The listing builds one solid part. Answer for the finished solid, in the listing's coordinates (mm). A direction names the side the tool comes from. Give positions to 0.01 mm unless a question says otherwise; leave off trailing zeros. Loops run counter-clockwise (first coordinate to the right, second up) from the corner with the lowest first, then second, coordinate; pieces in that order, holes last. Notation, with made-up numbers: (73.25, 88) -> (92.25, 88) arc R19 ccw to (92.25, 115) -> close; hole circle Ø2 at (22.25, 53). An arc over 180 degrees is marked (long way). One line per question, with ' | ' between items. Start each with the question number.
from build123d import *

# Parameters (mm, degrees)
CUT_EXTRUDE1_DEPTH = 35.421953112
FILLET1_R          = 0.635
FILLET2_R          = 2.032


with BuildPart() as part:
    # Sketch3 → Revolve1 (revolve)
    with BuildSketch(Plane(origin=(0, 0, 0), x_dir=(0, 0, -1), z_dir=(1, 0, 0)), mode=Mode.PRIVATE) as revolve1_sk:
        Polygon((6.4135, 0), (6.4135, -25.9842), (10.16, -25.9842), (10.16, -23.368), (15.9639, -23.368), (15.9639, 0), align=None)
    revolve(revolve1_sk.sketch.rotate(Axis((0, 17.16060519, 0), (0, -1, 0)), 180), axis=Axis((0, 17.16060519, 0), (0, -1, 0)))

    # Sketch2 → Cut-Extrude1 (cut, through all)
    with BuildSketch(Plane(origin=(0, 0, 0), x_dir=(1, 0, 0), z_dir=(0, 1, 0))):
        Polygon((7.405671903, 0), (3.702835951, 6.4135), (-3.702835951, 6.4135), (-7.405671903, 0), (-3.702835951, -6.4135), (3.702835951, -6.4135), align=None)
    extrude(amount=-CUT_EXTRUDE1_DEPTH, mode=Mode.SUBTRACT)

    # Fillet1
    fillet1_edges = [part.edges().sort_by_distance(p)[0] for p in [
        (5.554253927, -25.9842, -3.20675),
        (5.554253927, -25.9842, 3.20675),
        (0, -25.9842, -6.4135),
        (0, -25.9842, 6.4135),
        (-5.554253927, -25.9842, -3.20675),
        (-5.554253927, -25.9842, 3.20675),
        (0, 0, 6.4135),
        (-5.554253927, 0, 3.20675),
        (-5.554253927, 0, -3.20675),
        (0, 0, -6.4135),
        (5.554253927, 0, -3.20675),
        (5.554253927, 0, 3.20675),
        (0, 0, -15.9639),
        (0, -23.368, -15.9639),
        (0, -25.9842, -10.16),
    ]]
    fillet(fillet1_edges, radius=FILLET1_R)

    # Fillet2
    fillet2_edges = [part.edges().sort_by_distance(p)[0] for p in [
        (0, -23.368, -10.16),
    ]]
    fillet(fillet2_edges, radius=FILLET2_R)


solid = part.part
1. For faces 5 (the flat face through (0, -13, -6.414)), 6 (the flat face through (-5, -25.984, 6)), 7 (the cylindrical face through (5.7, -0.2, 3.3)), 8 (the cylindrical face through (5.68, -25.79, -3.35)), determine the directions among +Z, -Z, +X, -X, +Y, -Y from which every point of the face is accessible in a straight line to the end or side of a thin tool.
2. Determine the mould class of faces 1 (the cylindrical face through (5.74, -25.793, 3.248)), 2 (the flat face through (7, 0, 3)), 3 (the flat face through (-5.5, -12.8, -3.3)), 4 (the cylindrical face through (-4.795, -11.529, 15.227)) for opening direction X: released by +X, released by -X, zero draft, split by the parting line, or undercut.
3. The part is cut by section A-A (y = -12.25). Write down the section's boundary in (x, z), plus the area to 3 significant figures.
4. Each of these flat-tipped pins is pushed along its axis until it touches: pin 1 Ø4 at (x, y) = (10.5, -5) entering from +Z; pin 2 Ø3 at (y, z) = (-14.5, -5.5) entering from +X; pin 3 Ø1 at (x, y) = (7.5, -12.5) entering from +Z. Where does it stop, or does it pass through?
5. Straight lines are drawn through the part: L1, parallel to Y at x = 8, z = 11; L2, parallel to Z at x = -1, y = -1.5; L3, parallel to Z at x = -4.5, y = -9.75. For each, find the intervals that lie inside material, in ascending order.
Check sheet entries:
1) face 5: +Y, -Y | face 6: +Z, -Z, +X, -X, -Y | face 7: +Y | face 8: -Y
2) face 1: undercut | face 2: zero draft | face 3: undercut | face 4: split by the parting line
3) outline: circle Ø31.93 at (0, 0); hole (-7.41, 0) -> (-3.7, -6.41) -> (3.7, -6.41) -> (7.41, 0) -> (3.7, 6.41) -> (-3.7, 6.41) -> close | area: 658 mm^2
4) pin 1: stops at z = 13.51 | pin 2: stops at x = 15.45 | pin 3: stops at z = 14.35
5) L1: y = -23.37 to 0 | L2: z = -15.93 to -6.41, 6.41 to 15.93 | L3: z = -15.32 to -5.03, 5.03 to 15.32
